Source: three-view drawing plus pictorial views. Frame: mm from the lowest corner of the part. A direction names the side the tool comes from. Give positions to 0.01 mm unless a question says otherwise; leave off trailing zeros. Order: outer loops, then holes, each group sorted by start corner. A loop starts at its lowest first (then second) coordinate and runs counter-clockwise, first axis right, second up.
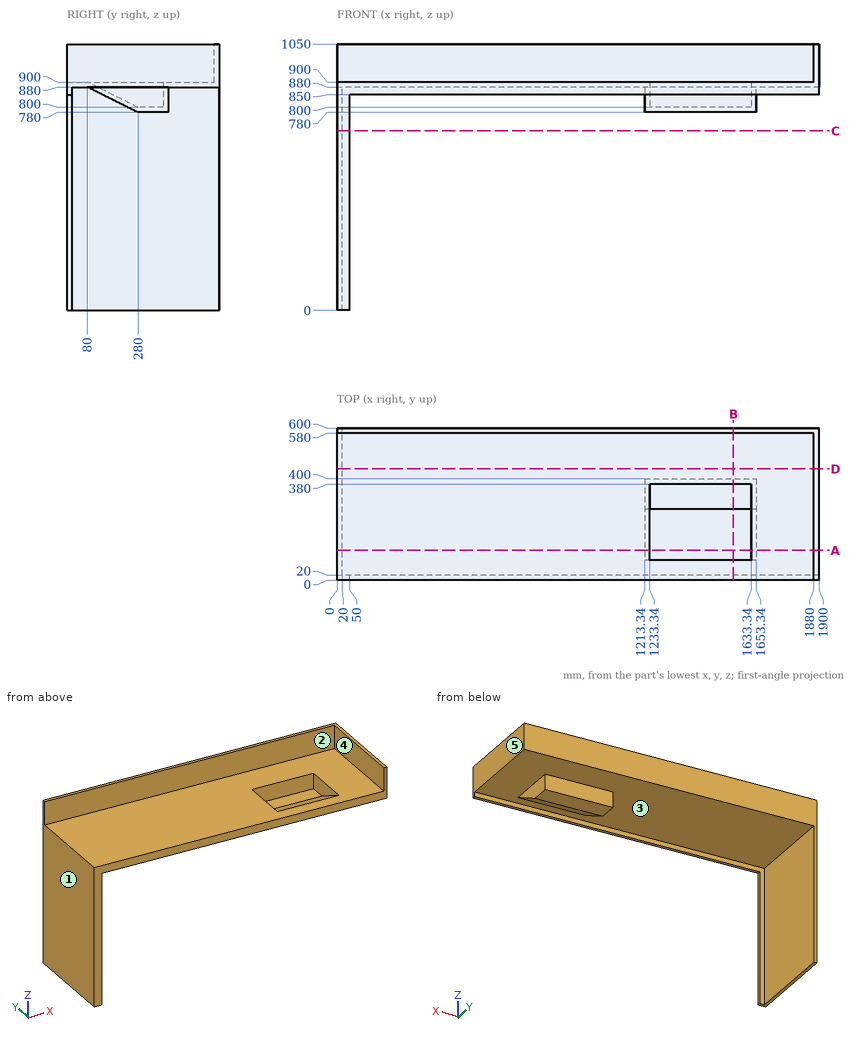
1) Section query B-B on x = 1562. Output: boundary loops of the cut face in (y, z).
Checks:
outline: (0, 850) - (20, 850) - (20, 880) - (80, 880) - (280, 780) - (400, 780) - (400, 880) - (600, 880) - (600, 1050) - (580, 1050) - (580, 900) - (380, 900) - (380, 800) - (280, 800) - (80, 900) - (0, 900) - close
2) Section query D-D on y = 439.5. Output: boundary loops of the cut face in (x, z), and give its area (3 significant figures).
Checks:
outline: (0, 0) - (20, 0) - (20, 880) - (1900, 880) - (1900, 1050) - (1880, 1050) - (1880, 900) - (0, 900) - close
area: 58,600 mm2
3) First-contact query: pin 1 Ø1.5 at (x, y) = (1044, 403) entering from +Z; pin 2 Ø1 at (y, z) = (352, 854) entering from +X; pin 3 Ø10 at (y, z) = (189.5, 435) entering from -X; pin 4 Ø4 at (x, y) = (1570, 188) entering from +Z. Flat tips, straight axial feed; report the tip coordinate or a pass-through.
Checks:
pin 1: stops at z = 900
pin 2: stops at x = 1653.34
pin 3: stops at x = 0
pin 4: stops at z = 847
4) Section query A-A on y = 119. Output: boundary loops of the cut face in (x, z).
Checks:
outline: (0, 0) - (20, 0) - (20, 880) - (1213.34, 880) - (1213.34, 860.5) - (1653.34, 860.5) - (1653.34, 880) - (1900, 880) - (1900, 1050) - (1880, 1050) - (1880, 900) - (1633.34, 900) - (1633.34, 880.5) - (1233.34, 880.5) - (1233.34, 900) - (0, 900) - close
5) Ray query, L1, parallel to Z at x = 1037, y = 435.5; L2, parallel to X at y = 156, z = 671; L3, parallel to Y at x = 1429.5, z = 819. Return the intervals inside material, ascending.
Checks:
L1: z = 880 to 900
L2: x = 0 to 20
L3: y = 202 to 242, 380 to 400
6) Reachability of the marked faces 4 and 5 from +Z, -Z, +X, -X, +Y, -Y: full face, straight path, thin tool, end or side. Return the list, or none.
Checks:
face 4: +Z, -X, -Y
face 5: +Z, -Z, +X, +Y, -Y
7) Pull-direction query (X, two-part tool) for the marked faces 1, 2 and 3; classes: +X half, -X half, draft (parallel to the pull), parting line (faces both ways), or undercut.
Checks:
face 1: -X half
face 2: draft
face 3: undercut
8) Section query C-C on z = 707. Output: boundary loops of the cut face in (x, y), and give its area (3 significant figures).
Checks:
outline: (0, 0) - (50, 0) - (50, 20) - (20, 20) - (20, 600) - (0, 600) - close
area: 12,600 mm2
